Verification items for this drawing (mm, ordinates from the low corner). A direction names the side the tool comes from. Round coordinates to 2 decimals unless told otherwise and drop trailing zeros. Order: outer loops, then holes, each group sorted by start corner. A loop starts at its lowest first (then second) coordinate and runs counter-clockwise, first axis right, second up. Notation, with made-up numbers: (-24.5, 49) -> (23.5, 49) arc R23 ccw to (23.5, 80) -> close; hole circle Ø10 at (-36, 25.25). An arc over 180 degrees is marked (long way). Answer in a Markdown table with one row per item. Add a question column.
1. Draft check along X on the marked faces 3, 4 and 5. Enter one of: +X half, -X half, draft (parallel to the pull), parting line (faces both ways), or undercut.
2. Sectioned sample at A-A, the plane y = 5. Record the boundary of the cut face in (x, z).
3. Access from +Z, -Z, +X, -X, +Y, -Y to the whole of each face (thin tool, end or side, straight path). Record for the marked faces 1 and 2.
4. Sectioned sample at C-C, the plane y = 14.75. Record the boundary of the cut face in (x, z), then the cut area to 3 significant figures.
5. Sectioned sample at B-B, the plane z = 6. Record the boundary of the cut face in (x, y).
6. Material ranges on L1, parallel to X at y = 7.25, z = 27; L2, parallel to Z at x = 30, y = 15, recorded low to high. Write a range as from..to.
7. Sectioned sample at D-D, the plane x = 20.5. Record the boundary of the cut face in (y, z), then the cut area to 3 significant figures.
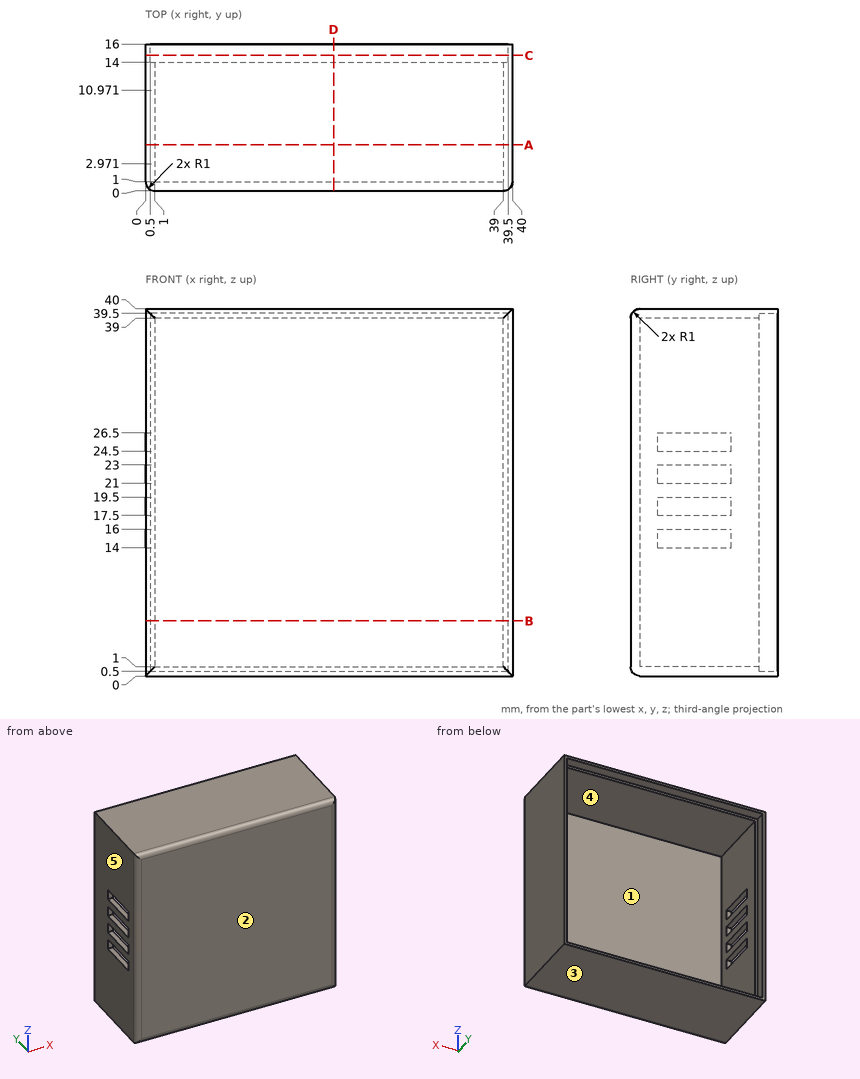
Answer key:
| question | item | result |
|---|---|---|
| 1 | face 3 | draft |
| 1 | face 4 | undercut |
| 1 | face 5 | -X half |
| 2 | outline | (0, 0) -> (40, 0) -> (40, 40) -> (0, 40) -> (0, 26.5) -> (1, 26.5) -> (1, 39) -> (39, 39) -> (39, 1) -> (1, 1) -> (1, 14) -> (0, 14) -> close; (0, 16) -> (1, 16) -> (1, 17.5) -> (0, 17.5) -> close; (0, 19.5) -> (1, 19.5) -> (1, 21) -> (0, 21) -> close; (0, 23) -> (1, 23) -> (1, 24.5) -> (0, 24.5) -> close |
| 3 | face 1 | +Y |
| 3 | face 2 | +Z, -Z, +X, -X, -Y |
| 4 | outline | (0, 0) -> (40, 0) -> (40, 40) -> (0, 40) -> close; hole (0.5, 0.5) -> (39.5, 0.5) -> (39.5, 39.5) -> (0.5, 39.5) -> close |
| 4 | area | 79.0 mm² |
| 5 | outline | (0, 1) arc R1 ccw to (1, 0) -> (39, 0) arc R1 ccw to (40, 1) -> (40, 16) -> (39.5, 16) -> (39.5, 14) -> (39, 14) -> (39, 1) -> (1, 1) -> (1, 14) -> (0.5, 14) -> (0.5, 16) -> (0, 16) -> close |
| 6 | L1 | x = 0..1, 39..40 |
| 6 | L2 | z = 0..0.5, 39.5..40 |
| 7 | outline | (0, 1) arc R1 ccw to (1, 0) -> (16, 0) -> (16, 0.5) -> (14, 0.5) -> (14, 1) -> (1, 1) -> (1, 39) -> (14, 39) -> (14, 39.5) -> (16, 39.5) -> (16, 40) -> (1, 40) arc R1 ccw to (0, 39) -> close |
| 7 | area | 67.6 mm² |
